Build history of the part. All positions in model axes, mm. Face numbers are marked on the shaded views. A direction names the side the tool comes from. Give positions to 0.01 mm unless a question says otherwise; leave off trailing zeros. Write each loop counter-clockwise with the first axis right and the second up, starting at its lowest first coordinate (ties: lowest second). Pieces come first, ordered by that corner, then holes. Notation, with made-up numbers: (51.25, 36) -> (98.25, 36) arc R19 cw to (98.25, 58) -> close; hole circle Ø9 at (12, -1.75). An arc over 180 degrees is marked (long way). Put each result on its own line as item: value.
from build123d import *

# Parameters (mm, degrees)
SKETCH1_R           = 77.724
BOSS_EXTRUDE1_DEPTH = 50.8
BOSS_EXTRUDE2_START = -50.8
BOSS_EXTRUDE2_DEPTH = 101.6
BOSS_EXTRUDE3_START = -50.8
SKETCH3_R           = 77.724
BOSS_EXTRUDE3_DEPTH = 101.6
CUT_EXTRUDE2_START  = -50.8
CUT_EXTRUDE2_DEPTH  = 967.835320745
CUT_EXTRUDE4_START  = -50.8
SKETCH5_R           = 76.2
CUT_EXTRUDE4_DEPTH  = 967.835320745
CUT_EXTRUDE6_START  = -50.8
SKETCH6_R           = 76.2
CUT_EXTRUDE6_DEPTH  = 967.835320745


with BuildPart() as part:
    # Sketch1 → Boss-Extrude1 (new, symmetric)
    with BuildSketch(Plane(origin=(0, 0, 0), x_dir=(1, 0, 0), z_dir=(0, 1, 0))):
        with Locations(Location((0, 0, 0), (0, 0, 270))):
            Circle(SKETCH1_R)
    extrude(amount=BOSS_EXTRUDE1_DEPTH, both=True)

    # Sketch2 → Boss-Extrude2 (add)
    with BuildSketch(Plane(origin=(0, 0, 0), x_dir=(1, 0, 0), z_dir=(0, 1, 0)).offset(BOSS_EXTRUDE2_START)):
        Polygon((-20.116451462, -75.075618922), (368.943803327, -179.324), (450.206196673, -179.324), (839.266451462, -75.075618922), (839.266451462, 75.075618922), (450.206196673, 179.324), (368.943803327, 179.324), (-20.116451462, 75.075618922), align=None)
    extrude(amount=BOSS_EXTRUDE2_DEPTH)

    # Sketch3 → Boss-Extrude3 (add)
    with BuildSketch(Plane(origin=(0, 0, 0), x_dir=(1, 0, 0), z_dir=(0, 1, 0)).offset(BOSS_EXTRUDE3_START)):
        with Locations((819.15, 0)):
            Circle(SKETCH3_R)
    extrude(amount=BOSS_EXTRUDE3_DEPTH)

    # Sketch4 → Cut-Extrude2 (cut, through all)
    with BuildSketch(Plane(origin=(0, 0, 0), x_dir=(1, 0, 0), z_dir=(0, 1, 0)).offset(CUT_EXTRUDE2_START)):
        Polygon((-19.722011237, -73.603547963), (369.144441733, -177.8), (450.005558267, -177.8), (838.872011237, -73.603547963), (838.872011237, 73.603547963), (450.005558267, 177.8), (369.144441733, 177.8), (-19.722011237, 73.603547963), align=None)
    extrude(amount=CUT_EXTRUDE2_DEPTH, mode=Mode.SUBTRACT)

    # Sketch5 → Cut-Extrude4 (cut, through all)
    with BuildSketch(Plane(origin=(0, 0, 0), x_dir=(1, 0, 0), z_dir=(0, 1, 0)).offset(CUT_EXTRUDE4_START)):
        Circle(SKETCH5_R)
    extrude(amount=CUT_EXTRUDE4_DEPTH, mode=Mode.SUBTRACT)

    # Sketch6 → Cut-Extrude6 (cut, through all)
    with BuildSketch(Plane(origin=(0, 0, 0), x_dir=(1, 0, 0), z_dir=(0, 1, 0)).offset(CUT_EXTRUDE6_START)):
        with Locations((819.15, 0)):
            Circle(SKETCH6_R)
    extrude(amount=CUT_EXTRUDE6_DEPTH, mode=Mode.SUBTRACT)


solid = part.part
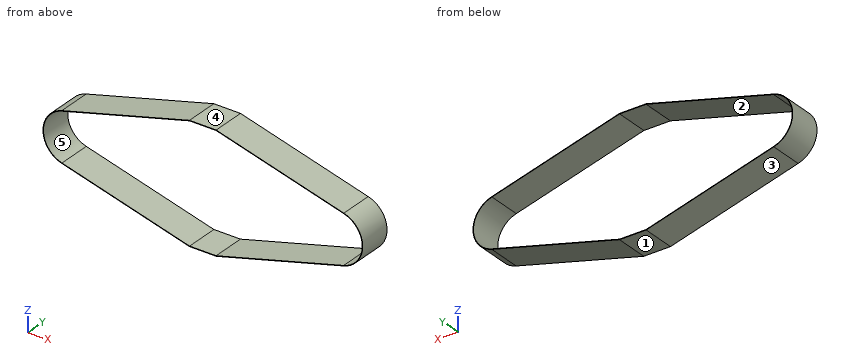
1) Pin check, flat tips, straight feed: pin 1 (3 mm diameter, centred on x = 156, y = -2.5, fed in from +Z); pin 2 (3 mm diameter, centred on y = -12, z = -73, fed in from +X); pin 3 (3 mm diameter, centred on y = -31, z = -19, fed in from -X). Stop position of each tip, or through.
Filled sheet:
pin 1: z = 122.67
pin 2: x = 849.63
pin 3: x = -75.73
2) Wall check: L1, parallel to Z at x = 641, y = 22; L2, parallel to Z at x = 530, y = 4.5; L3, parallel to X at y = 24.5, z = -21. Give the ranges that are in metal, low to high.
Filled sheet:
L1: -128.2 to -126.62, 126.62 to 128.2
L2: -157.94 to -156.37, 156.37 to 157.94
L3: -74.83 to -73.25, 892.4 to 893.98
3) Slice it at A-A (x = 83.5). Write the cut outline in (y, z), plus the area to 3 significant figures.
Filled sheet:
outline: (-50.8, -102.84) -> (50.8, -102.84) -> (50.8, -101.26) -> (-50.8, -101.26) -> close; (-50.8, 101.26) -> (50.8, 101.26) -> (50.8, 102.84) -> (-50.8, 102.84) -> close
area: 321 mm2
4) Pull direction X, two halves, no side cores. Call the marked faces 3, 4 and 5: released by +X, released by -X, zero draft, split by the parting line, or undercut.
Filled sheet:
face 3: released by -X
face 4: zero draft
face 5: undercut
5) Slice it at B-B (z = 50). Write the cut outline in (x, y).
Filled sheet:
outline: (-59.51, -50.8) -> (-57.5, -50.8) -> (-57.5, 50.8) -> (-59.51, 50.8) -> close; (876.65, -50.8) -> (878.66, -50.8) -> (878.66, 50.8) -> (876.65, 50.8) -> close
6) Tool access for the marked faces 1 and 2: list every direction of +Z, -Z, +X, -X, +Y, -Y with a clear straight run to the whole face (end or side of a thin tool).
Filled sheet:
face 1: -Z, +X, -X, +Y, -Y
face 2: +Y, -Y
7) Slice it at C-C (y = -6.5). Write the cut outline in (x, z), plus the area to 3 significant figures.
Filled sheet:
outline: (-20.12, -75.08) -> (368.94, -179.32) -> (450.21, -179.32) -> (839.27, -75.08) arc R77.72 ccw to (839.27, 75.08) -> (450.21, 179.32) -> (368.94, 179.32) -> (-20.12, 75.08) arc R77.72 ccw to start; hole (-19.72, -73.6) -> (369.14, -177.8) -> (450.01, -177.8) -> (838.87, -73.6) arc R76.2 ccw to (838.87, 73.6) -> (450.01, 177.8) -> (369.14, 177.8) -> (-19.72, 73.6) arc R76.2 ccw to start
area: 3,320 mm2
